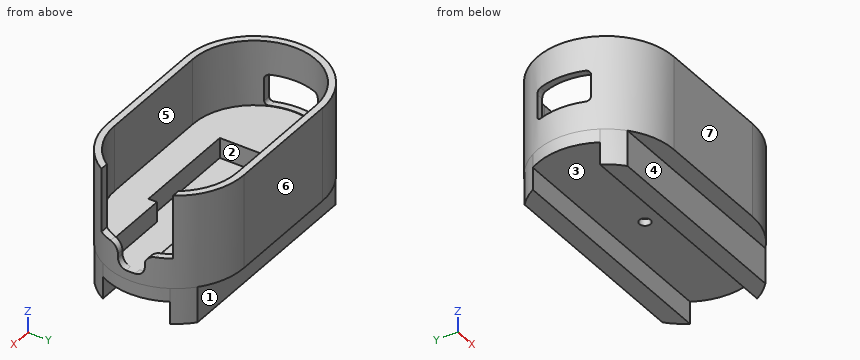
```python
from build123d import *

# Parameters (mm, degrees)
BOSS_EXTRUDE1_DEPTH = 19
BOSS_EXTRUDE2_DEPTH = 2
BOSS_EXTRUDE3_DEPTH = 4.5
SKETCH4_W           = 4.75
SKETCH4_H           = 6
SKETCH4_W_2         = 14.25
SKETCH4_H_2         = 16
CUT_EXTRUDE1_DEPTH  = 49.452157546
SKETCH5_W           = 7
SKETCH5_H           = 12
CUT_EXTRUDE2_DEPTH  = 49.452157546
FILLET1_R           = 1
SKETCH6_R           = 1.25
BOSS_EXTRUDE4_DEPTH = 3
BOSS_EXTRUDE7_DEPTH = 8
FILLET2_R           = 2
SKETCH9_R           = 1.252428217
CUT_EXTRUDE3_DEPTH  = 10
CUT_EXTRUDE6_START  = -1.5
CUT_EXTRUDE6_DEPTH  = 2.1


with BuildPart() as part:
    # Sketch1 → Boss-Extrude1 (new body)
    with BuildSketch(Plane.XY):
        with BuildLine():
            Line((-34.384444189, 18.719216619), (-7.984444189, 18.719216619))
            ThreePointArc((-7.984444189, 18.719216619), (7.265555811, 3.469216619), (-7.984444189, -11.780783381))
            Line((-7.984444189, -11.780783381), (-34.384444189, -11.780783381))
            ThreePointArc((-34.384444189, -11.780783381), (-49.634444189, 3.469216619), (-34.384444189, 18.719216619))
        make_face()
        with BuildLine():
            Line((-34.384444189, 17.219216619), (-7.984444189, 17.219216619))
            ThreePointArc((-7.984444189, 17.219216619), (5.765555811, 3.469216619), (-7.984444189, -10.280783381))
            Line((-7.984444189, -10.280783381), (-34.384444189, -10.280783381))
            ThreePointArc((-34.384444189, -10.280783381), (-48.134444189, 3.469216619), (-34.384444189, 17.219216619))
        make_face(mode=Mode.SUBTRACT)
    extrude(amount=BOSS_EXTRUDE1_DEPTH)



with BuildPart() as body_2:
    # Sketch2 → Boss-Extrude2 (new body)
    with BuildSketch(Plane(origin=(0, 0, 0), x_dir=(-1, 0, 0), z_dir=(0, 0, -1))):
        with BuildLine():
            Line((34.384444189, -11.780783381), (7.984444189, -11.780783381))
            ThreePointArc((7.984444189, -11.780783381), (-7.265555811, 3.469216619), (7.984444189, 18.719216619))
            Line((7.984444189, 18.719216619), (34.384444189, 18.719216619))
            ThreePointArc((34.384444189, 18.719216619), (49.634444189, 3.469216619), (34.384444189, -11.780783381))
        make_face()
    extrude(amount=BOSS_EXTRUDE2_DEPTH)


with BuildPart() as part_1:
    add(part.part)

    add(body_2.part)  # Boss-Extrude3 merges body 2
    # Sketch3 → Boss-Extrude3 (add)
    with BuildSketch(Plane.XY):
        with BuildLine():
            Line((-22.664695889, -3.430783381), (-33.184444189, -3.430783381))
            Line((-33.184444189, -3.430783381), (-33.184444189, 10.369216619))
            Line((-33.184444189, 10.369216619), (-19.704192488, 10.369216619))
            Line((-19.704192488, 10.369216619), (-9.184444189, 10.369216619))
            Line((-9.184444189, 10.369216619), (-9.184444189, 8.469216619))
            Line((-9.184444189, 8.469216619), (4.663184056, 8.469216619))
            ThreePointArc((4.663184056, 8.469216619), (-0.337155761, 14.715615149), (-7.984444189, 17.069308538))
            Line((-7.984444189, 17.069308538), (-34.384444189, 17.069308538))
            ThreePointArc((-34.384444189, 17.069308538), (-47.984536108, 3.469216619), (-34.384444189, -10.1308753))
            Line((-34.384444189, -10.1308753), (-7.984444189, -10.1308753))
            ThreePointArc((-7.984444189, -10.1308753), (-0.337155761, -7.777181911), (4.663184056, -1.530783381))
            Line((4.663184056, -1.530783381), (-9.184444189, -1.530783381))
            Line((-9.184444189, -1.530783381), (-9.184444189, -3.430783381))
            Line((-9.184444189, -3.430783381), (-19.704192488, -3.430783381))
            Line((-19.704192488, -3.430783381), (-22.664695889, -3.430783381))
        make_face()
    extrude(amount=BOSS_EXTRUDE3_DEPTH)

    # Sketch4 → Cut-Extrude1 (cut, through all)
    with BuildSketch(Plane.ZY.offset(9.184444189)):
        with Locations((2.375, 3.469216619)):
            Rectangle(SKETCH4_W, SKETCH4_H)
        with Locations((11.875, 3.469216619)):
            Rectangle(SKETCH4_W_2, SKETCH4_H_2)
    extrude(amount=-CUT_EXTRUDE1_DEPTH, mode=Mode.SUBTRACT)

    # Sketch5 → Cut-Extrude2 (cut, through all)
    with BuildSketch(Plane(origin=(-33.184444189, 0, 0), x_dir=(0, 0, -1), z_dir=(1, 0, 0))):
        with Locations((-8, 3.469216619)):
            Rectangle(SKETCH5_W, SKETCH5_H)
    extrude(amount=-CUT_EXTRUDE2_DEPTH, mode=Mode.SUBTRACT)

    # Fillet1
    fillet1_edges = [part_1.edges().sort_by_distance(p)[0] for p in [
        (-47.580403151, -2.530783381, 11.5),
        (-47.580403151, 9.469216619, 11.5),
        (-47.580403151, 9.469216619, 4.5),
        (-47.580403151, -2.530783381, 4.5),
    ]]
    fillet(fillet1_edges, radius=FILLET1_R)

    # Sketch6 → Boss-Extrude4 (add)
    with BuildSketch(Plane(origin=(0, 0, -2), x_dir=(-1, 0, 0), z_dir=(0, 0, -1))):
        with BuildLine():
            ThreePointArc((47.662715914, -4.030783381), (49.634444189, 3.469216619), (47.662715914, 10.969216619))
            Line((47.662715914, 10.969216619), (-5.293827536, 10.969216619))
            ThreePointArc((-5.293827536, 10.969216619), (-7.265555811, 3.469216619), (-5.293827536, -4.030783381))
            Line((-5.293827536, -4.030783381), (47.662715914, -4.030783381))
        make_face()
        with Locations((21.184444189, 3.469216619)):
            Circle(SKETCH6_R, mode=Mode.SUBTRACT)
    extrude(amount=BOSS_EXTRUDE4_DEPTH)

    # Sketch10 → Boss-Extrude7 (add)
    with BuildSketch(Plane(origin=(0, 0, -2), x_dir=(-1, 0, 0), z_dir=(0, 0, -1))):
        with BuildLine():
            Line((-5.293827536, -4.030783381), (47.662715914, -4.030783381))
            ThreePointArc((47.662715914, -4.030783381), (46.201857789, -6.169830834), (44.400057001, -8.030783381))
            Line((44.400057001, -8.030783381), (-2.031168623, -8.030783381))
            ThreePointArc((-2.031168623, -8.030783381), (-3.832969412, -6.169830834), (-5.293827536, -4.030783381))
        make_face()
        with BuildLine():
            Line((-5.293827536, 10.969216619), (47.662715914, 10.969216619))
            ThreePointArc((47.662715914, 10.969216619), (46.201857789, 13.108264072), (44.400057001, 14.969216619))
            Line((44.400057001, 14.969216619), (-2.031168623, 14.969216619))
            ThreePointArc((-2.031168623, 14.969216619), (-3.832969412, 13.108264072), (-5.293827536, 10.969216619))
        make_face()
    extrude(amount=BOSS_EXTRUDE7_DEPTH)

    # Fillet2
    fillet2_edges = [part_1.edges().sort_by_distance(p)[0] for p in [
        (6.200927538, 0.469216619, 0),
        (6.200927538, 6.469216619, 0),
        (6.200927538, 6.469216619, 4.75),
        (6.200927538, 0.469216619, 4.75),
    ]]
    fillet(fillet2_edges, radius=FILLET2_R)

    # Sketch9 → Cut-Extrude3 (cut)
    with BuildSketch(Plane(origin=(0, 0, -2), x_dir=(-1, 0, 0), z_dir=(0, 0, -1))):
        with Locations((21.184444189, 3.469216619)):
            Circle(SKETCH9_R)
    extrude(amount=-CUT_EXTRUDE3_DEPTH, mode=Mode.SUBTRACT)

    # Sketch13 → Cut-Extrude6 (cut)
    with BuildSketch(Plane(origin=(0, 0, -5), x_dir=(-1, 0, 0), z_dir=(0, 0, -1)).offset(CUT_EXTRUDE6_START)):
        Polygon((17.951282681, 3.469216619), (19.567863435, 0.669216619), (22.801024943, 0.669216619), (24.417605696, 3.469216619), (22.801024943, 6.269216619), (19.567863435, 6.269216619), align=None)
    extrude(amount=-CUT_EXTRUDE6_DEPTH, mode=Mode.SUBTRACT)


solid = part_1.part
```
Design review of the part built by this model. Coordinates are the model's own, in mm. Face numbers are marked on the shaded views. A direction names the side the tool comes from. Coordinates: 2 decimals unless noted, no trailing zeros. Order: outer loops, then holes, each group sorted by start corner. A loop starts at its lowest first (then second) coordinate and runs counter-clockwise, first axis right, second up.
1) Clearance check with flat-ended pins moving along their axes: pin 1 (1.5 mm diameter, centred on x = 4, y = -3.5, fed in from +Z); pin 2 (1.3 mm diameter, centred on x = -47.5, z = 7.5, fed in from -Y); pin 3 (1 mm diameter, centred on y = -2.5, z = 2.5, fed in from -X); pin 4 (1.7 mm diameter, centred on x = -21, z = -2.5, fed in from +Y). State where each tip first meets the part, or that it passes through.
2) Take a section at A-A, the plane z = -7.5. Give the boundary of the cut face in (x, y).
3) Wall thickness on line 1 along Y through (x, z) = (-33, 14.5); line 2 along Y through (x, z) = (-10.5, -6); line 3 along Y through (x, z) = (-4, 2.75): over which ranges is each line inside the solid? List them lowest first.
4) Take a section at C-C, the plane z = 12.25. Give the boundary of the cut face in (x, y), and give its area (3 significant figures).
5) Take a section at D-D, the plane z = 7. Give the boundary of the cut face in (x, y).
6) Take a section at B-B, the plane x = -11. Give the boundary of the cut face in (y, z).
7) Mouldability with a two-part tool opening along X and no side actions: class the marked faces 1 and 2 as +X half, -X half, draft (parallel to the pull), parting line (faces both ways), or undercut.
8) For the marked faces 3, 4, 5, 6 and 7, list the 3-axis set-ups (+Z, -Z, +X, -X, +Y, -Y) from which the entire face can be reached by the end or side of a thin tool; tool diameter is ignored.
Returned:
1. pin 1: stops at z = 4.75
1. pin 2: stops at y = -5.32
1. pin 3: stops at x = -48.62
1. pin 4: stops at y = 18.72
2. outline: (-47.66, -4.03) arc R15.25 ccw to (-44.4, -8.03) - (2.03, -8.03) arc R15.25 ccw to (5.29, -4.03) - close; (-47.66, 10.97) - (5.29, 10.97) arc R15.25 ccw to (2.03, 14.97) - (-44.4, 14.97) arc R15.25 ccw to start
3. line 1: y = -11.78 to -10.28, 17.22 to 18.72
3. line 2: y = -8.03 to -4.03, 10.97 to 14.97
3. line 3: y = -11.25 to -9.69, -9.53 to -1.53, 8.47 to 16.47, 16.63 to 18.19
4. outline: (-34.38, -11.78) - (-7.98, -11.78) arc R15.25 ccw to (5, -4.53) - (3.2, -4.53) arc R13.75 cw to (-7.98, -10.28) - (-34.38, -10.28) arc R13.75 cw to (-34.38, 17.22) - (-7.98, 17.22) arc R13.75 cw to (3.2, 11.47) - (5, 11.47) arc R15.25 ccw to (-7.98, 18.72) - (-34.38, 18.72) arc R15.25 ccw to start
4. area: 190 mm2
5. outline: (-48.4, -2.53) arc R15.25 ccw to (-34.38, -11.78) - (-7.98, -11.78) arc R15.25 ccw to (5, -4.53) - (3.2, -4.53) arc R13.75 cw to (-7.98, -10.28) - (-34.38, -10.28) arc R13.75 cw to (-46.76, -2.53) - close; (-48.4, 9.47) - (-46.76, 9.47) arc R13.75 cw to (-34.38, 17.22) - (-7.98, 17.22) arc R13.75 cw to (3.2, 11.47) - (5, 11.47) arc R15.25 ccw to (-7.98, 18.72) - (-34.38, 18.72) arc R15.25 ccw to start
6. outline: (-11.78, -2) - (-8.03, -2) - (-8.03, -10) - (-4.03, -10) - (-4.03, -5) - (10.97, -5) - (10.97, -10) - (14.97, -10) - (14.97, -2) - (18.72, -2) - (18.72, 19) - (17.22, 19) - (17.22, 0) - (17.07, 0) - (17.07, 4.5) - (10.37, 4.5) - (10.37, 0) - (-3.43, 0) - (-3.43, 4.5) - (-10.13, 4.5) - (-10.13, 0) - (-10.28, 0) - (-10.28, 19) - (-11.78, 19) - close
7. face 1: draft
7. face 2: undercut
8. face 3: -Z, +X, -X
8. face 4: -Z, +X, -X, -Y
8. face 5: +Z
8. face 6: +Z, -Z, +X, -X, +Y
8. face 7: +Z, -Z, +X, -X, -Y
